Work out the finished part from the listing and answer in its coordinate system (mm). A direction names the side the tool comes from. Round coordinates to 2 decimals unless told otherwise and drop trailing zeros. Order: outer loops, then holes, each group sorted by start corner. A loop starts at its lowest first (then second) coordinate and runs counter-clockwise, first axis right, second up. Notation, with made-up numbers: (-10.75, -38) - (11.25, -38) arc R27 cw to (11.25, -2) - close; hole circle Ø4 at (72.25, -16.75). An arc over 180 degrees is marked (long way). Answer in a Markdown table with one row per item.
from build123d import *

# Parameters (mm, degrees)
ESQUISSE1_W                     = 40.624989268
ESQUISSE1_H                     = 156.8
BOSS_EXTRU_1_DEPTH              = 4
ESQUISSE2_W                     = 9
ESQUISSE2_H                     = 156.8
BOSS_EXTRU_2_DEPTH              = 83.900004333
ESQUISSE3_W                     = 80.400004333
ESQUISSE3_H                     = 50
ENL_V_MAT_EXTRU_1_DEPTH         = 4
CONG_1_R                        = 5
D_GAGEMENT_M31_D                = 3.4
BOSS_EXTRU_3_DEPTH              = 4
ENL_V_MAT_EXTRU_2_DEPTH         = 156.924377041
ENL_V_MAT_EXTRU_3_DEPTH         = 160.236963297
TROU_TARAUD_M3X0_51_D           = 2.5
TROU_TARAUD_M4X0_71_D           = 3.3
R_P_TITION_LIN_AIRE1_COUNT      = 4
R_P_TITION_LIN_AIRE1_PITCH      = 25
R_P_TITION_LIN_AIRE1_COUNT_DIR2 = 3
R_P_TITION_LIN_AIRE1_PITCH_DIR2 = 25
D_GAGEMENT_M42_D                = 4.5
R_P_TITION_LIN_AIRE2_COUNT      = 3
R_P_TITION_LIN_AIRE2_PITCH      = 25
R_P_TITION_LIN_AIRE2_COUNT_DIR2 = 2
R_P_TITION_LIN_AIRE2_PITCH_DIR2 = 25
TROU_TARAUD_M4X0_72_D           = 3.3
SYM_TRIE2_COPY_1_D              = 3.3
SYM_TRIE2_COPY_2_D              = 3.3
SYM_TRIE2_COPY_3_D              = 3.3
SYM_TRIE2_COPY_4_D              = 3.3
SYM_TRIE2_COPY_5_D              = 3.3
SYM_TRIE2_COPY_6_D              = 3.3
SYM_TRIE2_COPY_7_D              = 3.3
SYM_TRIE2_COPY_8_D              = 3.3
SYM_TRIE2_COPY_9_D              = 3.3
SYM_TRIE2_COPY_10_D             = 4.5
SYM_TRIE2_COPY_11_D             = 4.5
SYM_TRIE2_COPY_12_D             = 4.5
SYM_TRIE2_COPY_13_D             = 4.5
SYM_TRIE2_COPY_14_D             = 4.5
CONG_2_R                        = 5


with BuildPart() as part:
    # Esquisse1 → Boss.-Extru.1 (new body)
    with BuildSketch(Plane.XY):
        with Locations((4.312505437, 50.7)):
            Rectangle(ESQUISSE1_W, ESQUISSE1_H)
    extrude(amount=BOSS_EXTRU_1_DEPTH)

    # Esquisse2 → Boss.-Extru.2 (add)
    with BuildSketch(Plane(origin=(0, 0, 0), x_dir=(-1, 0, 0), z_dir=(0, 0, -1))):
        with Locations((-20.125000071, 50.7)):
            Rectangle(ESQUISSE2_W, ESQUISSE2_H)
    extrude(amount=BOSS_EXTRU_2_DEPTH)

    # Esquisse3 → Enlèv. mat.-Extru.1 (cut)
    with BuildSketch(Plane.ZY.offset(-15.625000071)):
        with Locations((-43.700002166, 50.7)):
            Rectangle(ESQUISSE3_W, ESQUISSE3_H)
    extrude(amount=-ENL_V_MAT_EXTRU_1_DEPTH, mode=Mode.SUBTRACT)

    # Congé1
    cong_1_edges = [part.edges().sort_by_distance(p)[0] for p in [
        (17.625000071, 75.7, -3.5),
        (17.625000071, 25.7, -3.5),
    ]]
    fillet(cong_1_edges, radius=CONG_1_R)

    # Dégagement M31 (through all)
    with Locations(Plane.XY.offset(4)):
        with Locations((-10, -10), (-10, 10), (10, 10), (10, -10)):
            d_gagement_m31 = Hole(D_GAGEMENT_M31_D / 2)

    # Symétrie1: Dégagement M31 across plane
    add(d_gagement_m31.mirror(Plane.ZX.offset(50.7)), mode=Mode.SUBTRACT)

    # Esquisse8 → Boss.-Extru.3 (add)
    with BuildSketch(Plane(origin=(0, 129.1, 0), x_dir=(1, 0, 0), z_dir=(0, 1, 0))):
        Polygon((3.625000071, 0), (15.625000071, 12), (15.625000071, 0), align=None)
    boss_extru_3 = extrude(amount=-BOSS_EXTRU_3_DEPTH)

    # Esquisse10 → Enlèv. mat.-Extru.2 (cut, through all)
    with BuildSketch(Plane(origin=(0, 0, 0), x_dir=(-1, 0, 0), z_dir=(0, 0, -1))):
        Polygon((-3.625000071, 129.1), (15.999989197, 109.475010732), (15.999989197, 129.1), align=None)
    enl_v_mat_extru_2 = extrude(amount=-ENL_V_MAT_EXTRU_2_DEPTH, mode=Mode.SUBTRACT)

    # Esquisse11 → Enlèv. mat.-Extru.3 (cut, through all)
    with BuildSketch(Plane(origin=(24.625000071, 0, 0), x_dir=(0, 0, -1), z_dir=(1, 0, 0))):
        Polygon((83.900004333, 107.1), (12, 129.1), (83.900004333, 129.1), align=None)
    enl_v_mat_extru_3 = extrude(amount=-ENL_V_MAT_EXTRU_3_DEPTH, mode=Mode.SUBTRACT)

    # Trou taraudé M3x0.51 (through all)
    with Locations(Plane(origin=(24.625000071, 70.7, -71.970004333), x_dir=(0, 0, 1), z_dir=(1, 0, 0))):
        with Locations((0, 0), (0, 40), (55.94, 0), (55.94, 40)):
            Hole(TROU_TARAUD_M3X0_51_D / 2)

    # Trou taraudé M4x0.71 (through all)
    with Locations(Plane(origin=(24.625000071, 63.2, -2.25), x_dir=(0, 0, 1), z_dir=(1, 0, 0))):
        with Locations((0, 0)):
            trou_taraud_m4x0_71 = Hole(TROU_TARAUD_M4X0_71_D / 2)

    # Répétition linéaire1: Trou taraud_ M4x0.71 4 × 3, 2 skipped
    with Locations(*[(0, j * R_P_TITION_LIN_AIRE1_PITCH_DIR2, -i * R_P_TITION_LIN_AIRE1_PITCH) for i in range(R_P_TITION_LIN_AIRE1_COUNT) for j in range(R_P_TITION_LIN_AIRE1_COUNT_DIR2) if (i, j) not in ((0, 0), (2, 2), (3, 2))]):
        add(trou_taraud_m4x0_71, mode=Mode.SUBTRACT)

    # Dégagement M42 (through all)
    with Locations(Plane(origin=(24.625000071, 75.7, -14.75), x_dir=(0, 0, 1), z_dir=(1, 0, 0))):
        with Locations((0, 0)):
            d_gagement_m42 = Hole(D_GAGEMENT_M42_D / 2)

    # Répétition linéaire2: D_gagement M42 3 × 2
    with Locations(*[(0, j * R_P_TITION_LIN_AIRE2_PITCH_DIR2, -i * R_P_TITION_LIN_AIRE2_PITCH) for i in range(R_P_TITION_LIN_AIRE2_COUNT) for j in range(R_P_TITION_LIN_AIRE2_COUNT_DIR2) if (i, j) != (0, 0)]):
        add(d_gagement_m42, mode=Mode.SUBTRACT)

    # Trou taraudé M4x0.72 (through all)
    with Locations(Plane(origin=(24.625000071, 100.7, -77.25), x_dir=(0, 0, 1), z_dir=(1, 0, 0))):
        with Locations((0, 0)):
            trou_taraud_m4x0_72 = Hole(TROU_TARAUD_M4X0_72_D / 2)

    # Symétrie2: Boss.-Extru.3, Enlèv. mat.-Extru.2, Enlèv. mat.-Extru.3, Trou taraudé M4x0.71, Dégagement M42, Trou taraudé M4x0.72 across plane
    add(boss_extru_3.mirror(Plane.ZX.offset(50.7)))
    add(enl_v_mat_extru_2.mirror(Plane.ZX.offset(50.7)), mode=Mode.SUBTRACT)
    add(enl_v_mat_extru_3.mirror(Plane.ZX.offset(50.7)), mode=Mode.SUBTRACT)
    add(trou_taraud_m4x0_71.mirror(Plane.ZX.offset(50.7)), mode=Mode.SUBTRACT)
    add(d_gagement_m42.mirror(Plane.ZX.offset(50.7)), mode=Mode.SUBTRACT)
    add(trou_taraud_m4x0_72.mirror(Plane.ZX.offset(50.7)), mode=Mode.SUBTRACT)

    # Symétrie2 copy 1 (through all)
    with Locations(Plane(origin=(24.625000071, 13.2, -2.25), x_dir=(0, 0, 1), z_dir=(1, 0, 0))):
        with Locations((0, 0)):
            Hole(SYM_TRIE2_COPY_1_D / 2)

    # Symétrie2 copy 2 (through all)
    with Locations(Plane(origin=(24.625000071, -11.8, -2.25), x_dir=(0, 0, 1), z_dir=(1, 0, 0))):
        with Locations((0, 0)):
            Hole(SYM_TRIE2_COPY_2_D / 2)

    # Symétrie2 copy 3 (through all)
    with Locations(Plane(origin=(24.625000071, 38.2, -27.25), x_dir=(0, 0, 1), z_dir=(1, 0, 0))):
        with Locations((0, 0)):
            Hole(SYM_TRIE2_COPY_3_D / 2)

    # Symétrie2 copy 4 (through all)
    with Locations(Plane(origin=(24.625000071, 13.2, -27.25), x_dir=(0, 0, 1), z_dir=(1, 0, 0))):
        with Locations((0, 0)):
            Hole(SYM_TRIE2_COPY_4_D / 2)

    # Symétrie2 copy 5 (through all)
    with Locations(Plane(origin=(24.625000071, -11.8, -27.25), x_dir=(0, 0, 1), z_dir=(1, 0, 0))):
        with Locations((0, 0)):
            Hole(SYM_TRIE2_COPY_5_D / 2)

    # Symétrie2 copy 6 (through all)
    with Locations(Plane(origin=(24.625000071, 38.2, -52.25), x_dir=(0, 0, 1), z_dir=(1, 0, 0))):
        with Locations((0, 0)):
            Hole(SYM_TRIE2_COPY_6_D / 2)

    # Symétrie2 copy 7 (through all)
    with Locations(Plane(origin=(24.625000071, 13.2, -52.25), x_dir=(0, 0, 1), z_dir=(1, 0, 0))):
        with Locations((0, 0)):
            Hole(SYM_TRIE2_COPY_7_D / 2)

    # Symétrie2 copy 8 (through all)
    with Locations(Plane(origin=(24.625000071, 38.2, -77.25), x_dir=(0, 0, 1), z_dir=(1, 0, 0))):
        with Locations((0, 0)):
            Hole(SYM_TRIE2_COPY_8_D / 2)

    # Symétrie2 copy 9 (through all)
    with Locations(Plane(origin=(24.625000071, 13.2, -77.25), x_dir=(0, 0, 1), z_dir=(1, 0, 0))):
        with Locations((0, 0)):
            Hole(SYM_TRIE2_COPY_9_D / 2)

    # Symétrie2 copy 10 (through all)
    with Locations(Plane(origin=(24.625000071, 0.7, -14.75), x_dir=(0, 0, 1), z_dir=(1, 0, 0))):
        with Locations((0, 0)):
            Hole(SYM_TRIE2_COPY_10_D / 2)

    # Symétrie2 copy 11 (through all)
    with Locations(Plane(origin=(24.625000071, 25.7, -39.75), x_dir=(0, 0, 1), z_dir=(1, 0, 0))):
        with Locations((0, 0)):
            Hole(SYM_TRIE2_COPY_11_D / 2)

    # Symétrie2 copy 12 (through all)
    with Locations(Plane(origin=(24.625000071, 0.7, -39.75), x_dir=(0, 0, 1), z_dir=(1, 0, 0))):
        with Locations((0, 0)):
            Hole(SYM_TRIE2_COPY_12_D / 2)

    # Symétrie2 copy 13 (through all)
    with Locations(Plane(origin=(24.625000071, 25.7, -64.75), x_dir=(0, 0, 1), z_dir=(1, 0, 0))):
        with Locations((0, 0)):
            Hole(SYM_TRIE2_COPY_13_D / 2)

    # Symétrie2 copy 14 (through all)
    with Locations(Plane(origin=(24.625000071, 0.7, -64.75), x_dir=(0, 0, 1), z_dir=(1, 0, 0))):
        with Locations((0, 0)):
            Hole(SYM_TRIE2_COPY_14_D / 2)

    # Congé2
    cong_2_edges = [part.edges().sort_by_distance(p)[0] for p in [
        (20.125000071, 107.1, -83.900004333),
        (20.125000071, -5.7, -83.900004333),
    ]]
    fillet(cong_2_edges, radius=CONG_2_R)


solid = part.part
1) Each of these flat-tipped pins is pushed along its axis until it touches: pin 1 (3 mm diameter, centred on x = 17.5, z = -22.5, fed in from +Y); pin 2 (1.2 mm diameter, centred on x = 18, z = -78.5, fed in from -Y); pin 3 (8 mm diameter, centred on x = -2.5, y = 40, fed in from -Z); pin 4 (2 mm diameter, centred on y = 70.7, z = -16.03, fed in from +X). Where does it stop, or does it pass through?
Filled in:
| item | result |
|---|---|
| pin 1 | stops at y = 126.35 |
| pin 2 | stops at y = -7.54 |
| pin 3 | stops at z = 0 |
| pin 4 | passes through |
2) Which of the six approach directions +Z, -Z, +X, -X, +Y, -Y give full straight-line access (tool end or side, diameter ignored) to faces 1 (the face through (10.221, 89.714, 1.972)), 2 (the face through (18, 25.7, -27))?
Filled in:
| item | result |
|---|---|
| face 1 | +Z, -Z |
| face 2 | -Z, -X |
3) Find section C-C, the plane y = 10. Give the vertices of the cut face in (x, z) (3 decimals).
Filled in:
| item | result |
|---|---|
| outline | (-16, 0) - (-11.7, 0) - (-11.7, 4) - (-16, 4) - close; (-8.3, 0) - (8.3, 0) - (8.3, 4) - (-8.3, 4) - close; (11.7, 0) - (15.625, 0) - (15.625, -83.9) - (24.625, -83.9) - (24.625, 4) - (11.7, 4) - close |
4) Find section D-D, the plane z = -39.75. Give the vertices of the cut face in (x, y) (3 decimals), then the cut area to 3 significant figures.
Filled in:
| item | result |
|---|---|
| outline | (15.625, -19.209) - (24.625, -19.209) - (24.625, -1.55) - (15.625, -1.55) - close; (15.625, 2.95) - (24.625, 2.95) - (24.625, 23.45) - (15.625, 23.45) - close; (15.625, 77.95) - (24.625, 77.95) - (24.625, 98.45) - (15.625, 98.45) - close; (15.625, 102.95) - (24.625, 102.95) - (24.625, 120.609) - (15.625, 120.609) - close; (19.625, 27.95) - (24.625, 27.95) - (24.625, 73.45) - (19.625, 73.45) - close |
| area | 914 mm^2 |
5) Find section A-A, the plane y = 88.2. Give the vertices of the cut face in (x, z) (3 decimals).
Filled in:
| item | result |
|---|---|
| outline | (-16, 0) - (15.625, 0) - (15.625, -0.6) - (24.625, -0.6) - (24.625, 4) - (-16, 4) - close; (15.625, -83.9) - (24.625, -83.9) - (24.625, -78.9) - (15.625, -78.9) - close; (15.625, -75.6) - (24.625, -75.6) - (24.625, -53.9) - (15.625, -53.9) - close; (15.625, -50.6) - (24.625, -50.6) - (24.625, -28.9) - (15.625, -28.9) - close; (15.625, -25.6) - (24.625, -25.6) - (24.625, -3.9) - (15.625, -3.9) - close |
6) The mould has two halves that part along Z. Classify faces 3 (the face through (-9.779, 109.714, 1.972)), 4 (the face through (20.062, -4.939, -82.946)), 5 (the face through (20.062, 102.896, -14.262)): released by +Z, released by -Z, zero draft, split by the parting line, or undercut.
Filled in:
| item | result |
|---|---|
| face 3 | zero draft |
| face 4 | released by -Z |
| face 5 | undercut |
7) Find the intervals of material crossed by probe 1 along Z at (x, y) = (22.25, 100.7); probe 2 along Z at (x, y) = (18, 88); probe 3 along Y at (x, z) = (8.5, -1), in increasing order. Write a range as from..to.
Filled in:
| item | result |
|---|---|
| probe 1 | z = -83.9..-78.9, -75.6..-67, -62.5..-42, -37.5..-17, -12.5..4 |
| probe 2 | z = -83.9..-78.89, -75.61..-53.89, -50.61..-28.89, -25.61..-3.89, -0.61..4 |
| probe 3 | y = -27.7..-23.7, 125.1..129.1 |
8) Find section B-B, the plane x = 10. Give the vertices of the cut face in (y, z) (3 decimals).
Filled in:
| item | result |
|---|---|
| outline | (-27.7, -6.375) - (-23.7, -6.375) - (-23.7, 0) - (-11.7, 0) - (-11.7, 4) - (-27.7, 4) - close; (-8.3, 0) - (8.3, 0) - (8.3, 4) - (-8.3, 4) - close; (11.7, 0) - (89.7, 0) - (89.7, 4) - (11.7, 4) - close; (93.1, 0) - (109.7, 0) - (109.7, 4) - (93.1, 4) - close; (113.1, 0) - (125.1, 0) - (125.1, -6.375) - (129.1, -6.375) - (129.1, 4) - (113.1, 4) - close |
